Work out the finished part from the listing and answer in its coordinate system (mm). Face numbers are marked on the shaded views. A direction names the side the tool comes from. Give positions to 0.01 mm unless a question says otherwise; leave off trailing zeros. Loops run counter-clockwise (first coordinate to the right, second up) from the corner with the lowest first, then second, coordinate; pieces in that order, holes last. Notation, with made-up numbers: (-11.75, 64) - (5.25, 64) arc R22 cw to (5.25, 78) - close; hole circle Ø9 at (82, 9.5). An arc over 180 degrees is marked (long way). One line per item, written item: value.
from build123d import *

# Parameters (mm, degrees)
BOSS_EXTRUDE1_DEPTH     = 22
BOSS_EXTRUDE3_START     = -5
BOSS_EXTRUDE3_OUTLINE_R = 1.5
BOSS_EXTRUDE3_DEPTH     = 5
CHAMFER2_SIZE           = 1


# Read off the part's stored shape, not the designer's step: Boss-Extrude3
with BuildPart() as part:
    # Sketch1 → Boss-Extrude1 (new body)
    with BuildSketch(Plane(origin=(0, 0, 0), x_dir=(1, 0, 0), z_dir=(0, 1, 0))):
        with BuildLine():
            Line((0, -16.5), (0, -11.5))
            ThreePointArc((0, -11.5), (-8.131727984, -8.131727984), (-11.5, 0))
            Line((-11.5, 0), (-16.5, 0))
            Line((-16.5, 0), (-24.5, 0))
            Line((-24.5, 0), (-24.5, -5))
            Line((-24.5, -5), (-15.724185194, -5))
            ThreePointArc((-15.724185194, -5), (-9.740379869, -13.318220602), (0, -16.5))
        make_face()
        with BuildLine():
            Line((24.5, 0), (16.5, 0))
            Line((16.5, 0), (11.5, 0))
            ThreePointArc((11.5, 0), (8.131727984, -8.131727984), (0, -11.5))
            Line((0, -11.5), (0, -16.5))
            ThreePointArc((0, -16.5), (9.740379869, -13.318220602), (15.724185194, -5))
            Line((15.724185194, -5), (24.5, -5))
            Line((24.5, -5), (24.5, 0))
        make_face()
    extrude(amount=-BOSS_EXTRUDE1_DEPTH)

    # Boss-Extrude3 outline → Boss-Extrude3 (cut)
    with BuildSketch(Plane.XY.offset(5).offset(BOSS_EXTRUDE3_START)):
        with Locations((20.5, -18)):
            Circle(BOSS_EXTRUDE3_OUTLINE_R)
        with Locations((20.5, -4)):
            Circle(BOSS_EXTRUDE3_OUTLINE_R)
        with Locations((-20.5, -4)):
            Circle(BOSS_EXTRUDE3_OUTLINE_R)
        with Locations((-20.5, -18)):
            Circle(BOSS_EXTRUDE3_OUTLINE_R)
    extrude(amount=BOSS_EXTRUDE3_DEPTH, mode=Mode.SUBTRACT)

    # Chamfer2
    chamfer2_edges = [part.edges().sort_by_distance(p)[0] for p in [
        (-22, -18, 5),
        (19, -4, 5),
        (19, -18, 5),
        (-22, -4, 5),
    ]]
    chamfer(chamfer2_edges, length=CHAMFER2_SIZE)

    # Sketch4 → Cut-Revolve2 (revolve, cut)
    with BuildSketch(Plane(origin=(0, 0, 0), x_dir=(-1, 0, 0), z_dir=(0, 0, -1))):
        with BuildLine():
            Line((-11.5, 0), (-11.5, -6.5))
            ThreePointArc((-11.5, -6.5), (-12.947807153, -5.158599205), (-13.5, -3.263715381))
            Line((-13.5, -3.263715381), (-13.5, 0))
            Line((-13.5, 0), (-11.5, 0))
        make_face()
    revolve(axis=Axis((0, 2.834255205, 0), (0, -1, 0)), mode=Mode.SUBTRACT)


solid = part.part
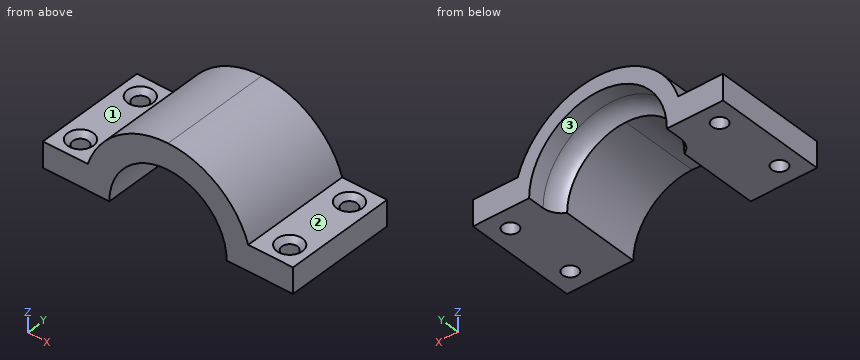
1. Section A-A (x = -20.5) is taken. Write down the section's boundary in (y, z).
Output:
outline: (-22, 0) - (-19.5, 0) - (-19.5, 4) - (-20.5, 5) - (-22, 5) - close; (-16.5, 0) - (-5.5, 0) - (-5.5, 4) - (-6.5, 5) - (-15.5, 5) - (-16.5, 4) - close; (-2.5, 0) - (0, 0) - (0, 5) - (-1.5, 5) - (-2.5, 4) - close
2. Section B-B (y = -4) is taken. Write down the section's boundary in (x, z).
Output:
outline: (-24.5, 0) - (-22, 0) - (-22, 4) - (-23, 5) - (-24.5, 5) - close; (-19, 0) - (-13.42, 0) arc R13.42 cw to (13.42, 0) - (19, 0) - (19, 4) - (18, 5) - (15.72, 5) arc R16.5 ccw to (-15.72, 5) - (-18, 5) - (-19, 4) - close; (22, 0) - (24.5, 0) - (24.5, 5) - (23, 5) - (22, 4) - close
3. Find the intervals of material crossed by line 1 along Y through (x, z) = (-20.5, 2.2); line 2 along Y through (x, z) = (-22, 4.75); line 3 along Z through (x, y) = (17, -2.75), in increasing order.
Output:
line 1: y = -22 to -19.5, -16.5 to -5.5, -2.5 to 0
line 2: y = -22 to -19.68, -16.32 to -5.68, -2.32 to 0
line 3: z = 0 to 5
4. Section D-D (y = -10.25) is taken. Write down the section's boundary in (x, z).
Output:
outline: (-24.5, 0) - (-11.5, 0) arc R11.5 cw to (11.5, 0) - (24.5, 0) - (24.5, 5) - (15.72, 5) arc R16.5 ccw to (-15.72, 5) - (-24.5, 5) - close
5. For the marked faces 1, 2 and 3, determine the directions among +Z, -Z, +X, -X, +Y, -Y from which every point of the face is accessible in a straight line to the end or side of a thin tool.
Output:
face 1: +Z, -X, +Y, -Y
face 2: +Z, +X, +Y, -Y
face 3: -Z, +Y
6. Flat-ended cylindrical pins translate along their axes: pin 1 Ø2.5 at (x, y) = (19, -14) entering from +Z; pin 2 Ø8 at (x, y) = (-5, -11) entering from +Z; pin 3 Ø4 at (x, y) = (-20.5, -4) entering from +Z. Find the tip coordinate at first contact, or state that the pin passes through.
Output:
pin 1: stops at z = 5
pin 2: stops at z = 16.47
pin 3: stops at z = 4.5
7. Section C-C (z = 2.5) is taken. Count the separate pieces of the cut face and the enclosed holes in it, and give its area (3 significant figures).
Output:
separate pieces: 2
enclosed holes: 4
area: 533 mm²
